Verification items for the finished model (mm, model axes). Face numbers are marked on the shaded views. A direction names the side the tool comes from. Round coordinates to 2 decimals unless told otherwise and drop trailing zeros. Write each loop counter-clockwise with the first axis right and the second up, starting at its lowest first coordinate (ties: lowest second). Pieces come first, ordered by that corner, then holes. Notation, with made-up numbers: M -31.5,-21.5 L 1.5,-21.5 A15 cw 1.5,-5.5 Z; hole C -22,-2 d1. An arc over 180 degrees is marked long. One line per item, written item: value. Start each with the question number.
Item 1: Section check A-A, the plane z = 23.5. Record the cut outline in (x, y), then the cut area to 3 significant figures.
Item 2: Tool access check on the marked faces 5, 6 and 7. Record the directions out of +Z, -Z, +X, -X, +Y, -Y that give a thin tool (end or side, any length) a straight path to the whole face; none if there is none.
Item 3: Draft check along Z on the marked faces 1, 2, 3 and 4. Enter one of: +Z half, -Z half, draft (parallel to the pull), parting line (faces both ways), or undercut.
Item 4: Section check D-D, the plane y = -20.5. Record the cut outline in (x, z), then the cut area to 3 significant figures.
Item 5: Section check B-B, the plane z = 63.5. Record the cut outline in (x, y).
Item 6: Section check C-C, the plane x = -13.5. Record the cut outline in (y, z), then the cut area to 3 significant figures.
Item 7: Thickness scan on probe 1 along Z at (x, y) = (5, -1); probe 2 along Z at (x, y) = (7.5, 2); probe 3 along Y at (x, z) = (9.5, -23). Record the ranges inside material, lowest first. Write a range as from..to.
Item 8: Gauge pin test, flat ends, axial feed: pin 1 (12 mm diameter, centred on y = 17.5, z = 17, fed in from +X); pin 2 (15.5 mm diameter, centred on x = 4, z = 36, fed in from -Y); pin 3 (18 mm diameter, centred on x = 0, z = -29.5, fed in from -Y); pin 4 (0.7 mm diameter, centred on y = 22, z = -41.5, fed in from +X). Record the tip position at first contact, or that the pin passes through.
from build123d import *

# Parameters (mm, degrees)
BOSS_EXTRUDE1_DEPTH = 9
SKETCH4_W           = 31
SKETCH4_H           = 8
SKETCH4_H_2         = 6
BOSS_EXTRUDE4_DEPTH = 45
CUT_EXTRUDE1_DEPTH  = 58
SKETCH6_3_R         = 11.25
CUT_EXTRUDE2_DEPTH  = 6
CUT_EXTRUDE3_DEPTH  = 4.3
CUT_EXTRUDE4_DEPTH  = 2.2
SKETCH9_3_R         = 4.65
CUT_EXTRUDE5_DEPTH  = 8
SKETCH10_W          = 31
SKETCH10_H          = 17
BOSS_EXTRUDE5_DEPTH = 59
SKETCH11_R          = 1.75
SKETCH11_W          = 21
SKETCH11_H          = 41
CUT_EXTRUDE6_DEPTH  = 38
SKETCH13_W          = 14
SKETCH13_H          = 5
CUT_EXTRUDE8_DEPTH  = 9


with BuildPart() as part:
    # Sketch1 → Boss-Extrude1 (new body)
    with BuildSketch(Plane.XY):
        Polygon((15.5, -28.5), (-15.5, -28.5), (-15.5, -10.3), (-15.5, 10.3), (-15.5, 28.5), (15.5, 28.5), align=None)
    extrude(amount=BOSS_EXTRUDE1_DEPTH)

    # Sketch4 → Boss-Extrude4 (add)
    with BuildSketch(Plane(origin=(0, 0, 0), x_dir=(-1, 0, 0), z_dir=(0, 0, -1))):
        with Locations((0, 24.5)):
            Rectangle(SKETCH4_W, SKETCH4_H)
        with Locations((0, -25.5)):
            Rectangle(SKETCH4_W, SKETCH4_H_2)
    extrude(amount=BOSS_EXTRUDE4_DEPTH)

    # Sketch6 → Cut-Extrude1 (cut, through all)
    with BuildSketch(Plane.XZ.offset(28.5)):
        with BuildLine():
            ThreePointArc((15.5, -29.5), (10.960155101, -40.460155116), (-2.1e-08, -45))
            Line((-2.1e-08, -45), (15.5, -45))
            Line((15.5, -45), (15.5, -29.5))
        make_face()
        with BuildLine():
            ThreePointArc((-2.1e-08, -45), (-10.960155116, -40.460155101), (-15.5, -29.5))
            Line((-15.5, -29.5), (-15.5, -45))
            Line((-15.5, -45), (-2.1e-08, -45))
        make_face()
    extrude(amount=-CUT_EXTRUDE1_DEPTH, mode=Mode.SUBTRACT)

    # Sketch6<3> → Cut-Extrude2 (cut)
    with BuildSketch(Plane.XZ.offset(28.5)):
        with Locations((0, -29.5)):
            Circle(SKETCH6_3_R)
    extrude(amount=-CUT_EXTRUDE2_DEPTH, mode=Mode.SUBTRACT)

    # Sketch7 → Cut-Extrude3 (cut)
    with BuildSketch(Plane(origin=(0, 28.5, 0), x_dir=(1, 0, 0), z_dir=(0, 1, 0))):
        with BuildLine():
            Line((-17.1, 31.65), (-4.313351365, 33.813351365))
            Line((-4.313351365, 33.813351365), (-2.15, 46.6))
            ThreePointArc((-2.15, 46.6), (0, 48.75), (2.15, 46.6))
            Line((2.15, 46.6), (4.313351365, 33.813351365))
            Line((4.313351365, 33.813351365), (17.1, 31.65))
            ThreePointArc((17.1, 31.65), (19.25, 29.5), (17.1, 27.35))
            Line((17.1, 27.35), (4.313351365, 25.186648635))
            Line((4.313351365, 25.186648635), (2.15, 12.4))
            ThreePointArc((2.15, 12.4), (0, 10.25), (-2.15, 12.4))
            Line((-2.15, 12.4), (-4.313351365, 25.186648635))
            Line((-4.313351365, 25.186648635), (-17.1, 27.35))
            ThreePointArc((-17.1, 27.35), (-19.25, 29.5), (-17.1, 31.65))
        make_face()
    extrude(amount=-CUT_EXTRUDE3_DEPTH, mode=Mode.SUBTRACT)

    # Sketch9 → Cut-Extrude4 (cut)
    with BuildSketch(Plane.XZ.offset(-20.5)):
        with BuildLine():
            ThreePointArc((3.25, -32.82565783), (0, -34.15), (-3.25, -32.82565783))
            Line((-3.25, -32.82565783), (-3.25, -44.655444566))
            ThreePointArc((-3.25, -44.655444566), (0, -45), (3.25, -44.655444566))
            Line((3.25, -44.655444566), (3.25, -32.82565783))
        make_face()
    extrude(amount=-CUT_EXTRUDE4_DEPTH, mode=Mode.SUBTRACT)

    # Sketch9<3> → Cut-Extrude5 (cut)
    with BuildSketch(Plane.XZ.offset(-20.5)):
        with Locations((0, -29.5)):
            Circle(SKETCH9_3_R)
    extrude(amount=-CUT_EXTRUDE5_DEPTH, mode=Mode.SUBTRACT)

    # Sketch10 → Boss-Extrude5 (add)
    with BuildSketch(Plane.XY.offset(9)):
        Rectangle(SKETCH10_W, SKETCH10_H)
    extrude(amount=BOSS_EXTRUDE5_DEPTH)

    # Sketch11 → Cut-Extrude6 (cut, through all)
    with BuildSketch(Plane.XZ.offset(8.5)):
        with Locations((5.2, 13.5)):
            Circle(SKETCH11_R)
        with Locations((-5.2, 13.5)):
            Circle(SKETCH11_R)
        with Locations((5.2, 63.5)):
            Circle(SKETCH11_R)
        with Locations((-5.2, 63.5)):
            Circle(SKETCH11_R)
        with Locations((0, 38.5)):
            Rectangle(SKETCH11_W, SKETCH11_H)
    extrude(amount=-CUT_EXTRUDE6_DEPTH, mode=Mode.SUBTRACT)

    # Sketch13 → Cut-Extrude8 (cut)
    with BuildSketch(Plane(origin=(0, 28.5, 0), x_dir=(1, 0, 0), z_dir=(0, 1, 0))):
        with Locations((0, 3.5)):
            Rectangle(SKETCH13_W, SKETCH13_H)
    extrude(amount=-CUT_EXTRUDE8_DEPTH, mode=Mode.SUBTRACT)


solid = part.part
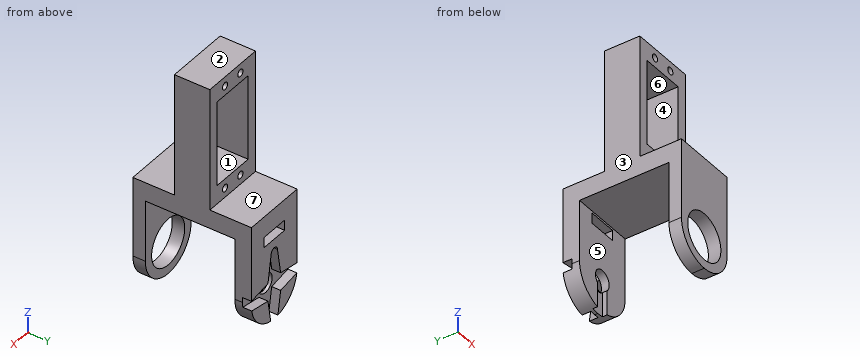
Response values:
1. outline: M -15.5,-8.5 L -10.5,-8.5 L -10.5,8.5 L -15.5,8.5 Z; M 10.5,-8.5 L 15.5,-8.5 L 15.5,8.5 L 10.5,8.5 Z
1. area: 170 mm2
2. face 5: -Z, +X, -X
2. face 6: +Y, -Y
2. face 7: +Z, +X, -X, +Y
3. face 1: undercut
3. face 2: +Z half
3. face 3: draft
3. face 4: undercut
4. outline: M -15.5,0 L 15.5,0 L 15.5,9 L -15.5,9 Z
4. area: 279 mm2
5. outline: M -15.5,-8.5 L -6.95,-8.5 L -6.95,8.5 L -15.5,8.5 Z; M -3.45,-8.5 L 3.45,-8.5 L 3.45,8.5 L -3.45,8.5 Z; M 6.95,-8.5 L 15.5,-8.5 L 15.5,8.5 L 6.95,8.5 Z
6. outline: M -28.5,-37.12 L -22.5,-37.12 L -22.5,0 L 20.5,0 L 20.5,-37.12 L 28.5,-37.12 L 28.5,-32.26 L 24.2,-32.26 L 24.2,-26.74 L 28.5,-26.74 L 28.5,9 L 8.5,9 L 8.5,68 L -8.5,68 L -8.5,9 L -28.5,9 Z
6. area: 2,010 mm2
7. probe 1: z = 0..11.76, 15.24..18, 59..61.76, 65.24..68
7. probe 2: z = 0..18, 59..68
7. probe 3: y = -28.5..-22.5, 20.5..28.5
8. pin 1: passes through
8. pin 2: stops at y = -8.5
8. pin 3: stops at y = 20.5
8. pin 4: stops at x = 10.22
